from build123d import *

# Parameters (mm, degrees)
SKETCH1_R               = 1.2065
SKETCH1_R_2             = 1.0795
BOSS_EXTRUDE1_DEPTH     = 10
CUT_EXTRUDE4_DEPTH      = 10
CUT_EXTRUDE4_DEPTH_BACK = 10
SKETCH6_R               = 0.2
CUT_EXTRUDE5_DEPTH      = 10
CUT_EXTRUDE5_DEPTH_BACK = 10


with BuildPart() as part:
    # Sketch1 → Boss-Extrude1 (new body)
    with BuildSketch(Plane(origin=(0, 0, 0), x_dir=(0, 0, -1), z_dir=(1, 0, 0))):
        Circle(SKETCH1_R)
        Circle(SKETCH1_R_2, mode=Mode.SUBTRACT)
    extrude(amount=BOSS_EXTRUDE1_DEPTH)

    # Sketch5 → Cut-Extrude4 (cut, two sides)
    with BuildSketch(Plane.XY) as cut_extrude4_sk:
        with BuildLine():
            Line((1.013670485, 0.9921875), (0, 0.9921875))
            Line((0, 0.9921875), (0, -0.9921875))
            Line((0, -0.9921875), (1.013670485, -0.9921875))
            ThreePointArc((1.013670485, -0.9921875), (2.005857985, 0), (1.013670485, 0.9921875))
        make_face()
    extrude(amount=CUT_EXTRUDE4_DEPTH, mode=Mode.SUBTRACT)
    extrude(cut_extrude4_sk.sketch, amount=-CUT_EXTRUDE4_DEPTH_BACK, mode=Mode.SUBTRACT)

    # Sketch6 → Cut-Extrude5 (cut, two sides)
    with BuildSketch(Plane(origin=(0, 0, 0), x_dir=(1, 0, 0), z_dir=(0, 1, 0))) as cut_extrude5_sk:
        with Locations((1.255857985, 0)):
            Circle(SKETCH6_R)
    extrude(amount=CUT_EXTRUDE5_DEPTH, mode=Mode.SUBTRACT)
    extrude(cut_extrude5_sk.sketch, amount=-CUT_EXTRUDE5_DEPTH_BACK, mode=Mode.SUBTRACT)


solid = part.part
The listing builds one solid part. Answer for the finished solid, in the listing's coordinates (mm). Give positions to 0.01 mm unless a question says otherwise; leave off trailing zeros. Write each loop counter-clockwise with the first axis right and the second up, starting at its lowest first coordinate (ties: lowest second). Pieces come first, ordered by that corner, then holes. Notation, with made-up numbers: (-39.5, 75) - (0.5, 75) arc R27 ccw to (0.5, 103) - close; hole circle Ø5 at (-20.5, 67.5). An arc over 180 degrees is marked (long way). One line per question, with ' | ' between items. Start each with the question number.
1. Section C-C, the plane z = -0.85 is taken. Determine the outline of the cut face in (x, y), then the cut area to 3 significant figures.
2. Section B-B, the plane z = 0 is taken. Determine the outline of the cut face in (x, y), then the cut area to 3 significant figures.
3. Given P1, Ø1, axis at x = 7, y = -0.5, coming from the -Z side, flat-ended and moving along its own axis, determine where the tip first touches the part or whether it passes through.
4. Section A-A, the plane y = 0 is taken. Determine the outline of the cut face in (x, z), then the cut area to 3 significant figures.
5. Section D-D, the plane x = 8 is taken. Determine the outline of the cut face in (y, z), then the cut area to 3 significant figures.
6. Straight lines are drawn through the part: line 1 (X direction, y = 1.15, z = 0); line 2 (Z direction, x = 6.75, y = 0.7); line 3 (Y direction, x = 8, z = 0.65). For each, find the intervals that lie inside material, in ascending order.
Result:
1) outline: (1.51, -0.86) - (10, -0.86) - (10, -0.67) - (1.75, -0.67) arc R0.99 cw to start; (1.51, 0.86) arc R0.99 cw to (1.75, 0.67) - (10, 0.67) - (10, 0.86) - close | area: 3.19 mm2
2) outline: (0, -1.21) - (1.06, -1.21) - (1.06, -1.08) - (0, -1.08) - close; (0, 1.08) - (1.06, 1.08) - (1.06, 1.21) - (0, 1.21) - close; (1.46, -1.21) - (10, -1.21) - (10, -1.08) - (1.46, -1.08) - close; (1.46, 1.08) - (10, 1.08) - (10, 1.21) - (1.46, 1.21) - close | area: 2.44 mm2
3) P1: stops at z = -1.21
4) outline: (2.01, -1.21) - (10, -1.21) - (10, -1.08) - (2.01, -1.08) - close; (2.01, 1.08) - (10, 1.08) - (10, 1.21) - (2.01, 1.21) - close | area: 2.03 mm2
5) outline: circle Ø2.41 at (0, 0); hole circle Ø2.16 at (0, 0) | area: 0.912 mm2
6) line 1: x = 0 to 1.06, 1.46 to 10 | line 2: z = -0.98 to -0.82, 0.82 to 0.98 | line 3: y = -1.02 to -0.86, 0.86 to 1.02
